The listing builds one solid part. Answer for the finished solid, in the listing's coordinates (mm). A direction names the side the tool comes from. Give positions to 0.01 mm unless a question says otherwise; leave off trailing zeros. Loops run counter-clockwise (first coordinate to the right, second up) from the corner with the lowest first, then second, coordinate; pieces in that order, holes last. Notation, with made-up numbers: (82, 16) - (116, 16) arc R35 cw to (116, 53) - close; hole circle Ø3 at (63.25, 89). An arc over 180 degrees is marked (long way). Write each question's results on one line, items separated by ' | '.
from build123d import *

# Parameters (mm, degrees)
F0_W     = 36
F0_H     = 36
F0_R     = 1.5
F1_DEPTH = 1.6
F2_R     = 2
F3_R     = 1.5
F4_DEPTH = 25
F6_DEPTH = 25
F7_R     = 1


with BuildPart() as f1:
    # F0 (on Top) → F1 (new body)
    with BuildSketch(Plane.XY):
        with Locations((18, 18)):
            Rectangle(F0_W, F0_H)
        with Locations((2.75, 2.75)):
            Circle(F0_R, mode=Mode.SUBTRACT)
        with Locations((33.25, 2.75)):
            Circle(F0_R, mode=Mode.SUBTRACT)
        with Locations((2.75, 33.25)):
            Circle(F0_R, mode=Mode.SUBTRACT)
        with Locations((33.25, 33.25)):
            Circle(F0_R, mode=Mode.SUBTRACT)
    extrude(amount=F1_DEPTH)

    # F2
    f2_edges = [f1.edges().sort_by_distance(p)[0] for p in [
        (0, 36, 0.8),
        (36, 36, 0.8),
        (36, 0, 0.8),
        (0, 0, 0.8),
    ]]
    fillet(f2_edges, radius=F2_R)

    # F3 (on face) → F4 (cut)
    with BuildSketch(Plane.XY.offset(1.6)):
        with Locations((8, 28)):
            Circle(F3_R)
        with Locations((8, 8)):
            Circle(F3_R)
        with Locations((28, 28)):
            Circle(F3_R)
        with Locations((28, 8)):
            Circle(F3_R)
    extrude(amount=-F4_DEPTH, mode=Mode.SUBTRACT)

    # F5 (on face) → F6 (cut)
    with BuildSketch(Plane.XY.offset(1.6)):
        Polygon((11, 5), (25, 5), (25, 11), (31, 11), (31, 25), (25, 25), (25, 31), (11, 31), (11, 25), (5, 25), (5, 11), (11, 11), align=None)
    extrude(amount=-F6_DEPTH, mode=Mode.SUBTRACT)

    # F7
    f7_edges = [f1.edges().sort_by_distance(p)[0] for p in [
        (11, 25, 0.8),
        (25, 25, 0.8),
        (25, 11, 0.8),
        (11, 11, 0.8),
        (11, 5, 0.8),
        (5, 11, 0.8),
        (25, 5, 0.8),
        (31, 11, 0.8),
        (5, 25, 0.8),
        (11, 31, 0.8),
        (31, 25, 0.8),
        (25, 31, 0.8),
    ]]
    fillet(f7_edges, radius=F7_R)


solid = f1.part
Item 1: A cutting plane is placed at B-B, the plane x = 28. Determine the outline of the cut face in (y, z), plus the area to 3 significant figures.
Values found:
outline: (0, 0) - (6.5, 0) - (6.5, 1.6) - (0, 1.6) - close; (9.5, 0) - (11, 0) - (11, 1.6) - (9.5, 1.6) - close; (25, 0) - (26.5, 0) - (26.5, 1.6) - (25, 1.6) - close; (29.5, 0) - (36, 0) - (36, 1.6) - (29.5, 1.6) - close | area: 25.6 mm²
Item 2: Find the intervals of material crossed by line 1 along Y through (x, z) = (2.75, 0.9); line 2 along Y through (x, z) = (28, 0.9); line 3 along Y through (x, z) = (27, 0.7), in increasing order. Write a range as [from, to].
Values found:
line 1: y = [0, 1.25], [4.25, 31.75], [34.75, 36] | line 2: y = [0, 6.5], [9.5, 11], [25, 26.5], [29.5, 36] | line 3: y = [0, 6.88], [9.12, 11], [25, 26.88], [29.12, 36]
Item 3: A cutting plane is placed at A-A, the plane y = 15.5. Determine the outline of the cut face in (x, z).
Values found:
outline: (0, 0) - (5, 0) - (5, 1.6) - (0, 1.6) - close; (31, 0) - (36, 0) - (36, 1.6) - (31, 1.6) - close
Item 4: A flat-ended cylindrical pin translates along its axis: P1, Ø1.8, axis at x = 8, y = 28, coming from the -Z side. Find the tip coordinate at first contact, or state that the pin passes through.
Values found:
P1: passes through
Item 5: For faces 4 (the face through (0.57, 35.4, 0.81)), 5 (the face through (10.715, 25.301, 0.789)), determine the directions among +Z, -Z, +X, -X, +Y, -Y from which every point of the face is accessible in a straight line to the end or side of a thin tool.
Values found:
face 4: +Z, -Z, -X, +Y | face 5: +Z, -Z
Item 6: A cutting plane is placed at C-C, the plane y = 2.75. Determine the outline of the cut face in (x, z), plus the area to 3 significant figures.
Values found:
outline: (0, 0) - (1.25, 0) - (1.25, 1.6) - (0, 1.6) - close; (4.25, 0) - (31.75, 0) - (31.75, 1.6) - (4.25, 1.6) - close; (34.75, 0) - (36, 0) - (36, 1.6) - (34.75, 1.6) - close | area: 48.0 mm²
Item 7: For a pull along Y with two mould halves and no side action, classify faces 1 (the face through (25.285, 10.699, 0.789)), 2 (the face through (18, 36, 1)), 3 (the face through (35.4, 0.57, 0.81)) as released by +Y, released by -Y, zero draft, split by the parting line, or undercut.
Values found:
face 1: undercut | face 2: released by +Y | face 3: released by -Y
